```python
from build123d import *

# Parameters (mm, degrees)
F0_R      = 30
F0_R_2    = 1.55
F0_W      = 15
F0_H      = 3.2
F1_DEPTH  = 7
F3_R      = 1.6
F4_DEPTH  = 3.5
F7_COUNT  = 3
F8_R      = 5
F9_DEPTH  = 25
F11_DEPTH = 5


with BuildPart() as f1:
    # F0 (on Top) → F1 (new body)
    with BuildSketch(Plane.XY):
        Circle(F0_R)
        Polygon((-4.1143593539, -10.3262794416), (-11.6143593539, -23.3166604984), (-14.3856406461, -21.7166604984), (-6.8856406461, -8.7262794416), align=None, mode=Mode.SUBTRACT)
        with Locations((13, -22.5166604984)):
            Circle(F0_R_2, mode=Mode.SUBTRACT)
        with Locations((-26, 0)):
            Circle(F0_R_2, mode=Mode.SUBTRACT)
        Polygon((-6.8856406461, 8.7262794416), (-14.3856406461, 21.7166604984), (-11.6143593539, 23.3166604984), (-4.1143593539, 10.3262794416), align=None, mode=Mode.SUBTRACT)
        with Locations((18.5, 0)):
            Rectangle(F0_W, F0_H, mode=Mode.SUBTRACT)
        with Locations((13, 22.5166604984)):
            Circle(F0_R_2, mode=Mode.SUBTRACT)
    extrude(amount=F1_DEPTH)

    # F3 (on offset) → F4 (join)
    with BuildSketch(Plane.XZ.offset(1.6)):
        Polygon((11, 7), (26, 7), (26, 12), (23.5, 12.5), (13.5, 12.5), (11, 12), align=None)
        with Locations((18.5, 9.5)):
            Circle(F3_R, mode=Mode.SUBTRACT)
    extrude(amount=F4_DEPTH)

    # F5: F1 across plane


with BuildPart() as f1_1:
    add(f1.part)
    add(f1.part.mirror(Plane.XZ))

    # F7: F1 ×3 about axis
    f7_axis = Axis((0, 0, 17.4874160439), (0, 0, 1))


with BuildPart() as f1_2:
    add(f1_1.part)
    for i in range(1, F7_COUNT):
        add(f1_1.part.rotate(f7_axis, i * 360 / F7_COUNT))

    # F8 (on face) → F9 (cut)
    with BuildSketch(Plane.XY.offset(7)):
        Circle(F8_R)
    extrude(amount=-F9_DEPTH, mode=Mode.SUBTRACT)

    # F10 (on face) → F11 (cut)
    with BuildSketch(Plane.XY.offset(7)):
        Polygon((-30, 5), (-30, 0), (-30, -5), (-23, -5), (-23, 0), (-23, 5), align=None)
        Polygon((11.5, -19.918584287), (7.1698729811, -22.418584287), (10.6698729811, -28.4807621135), (15, -25.9807621135), (19.3301270189, -23.4807621135), (15.8301270189, -17.418584287), align=None)
        Polygon((11.5, 19.918584287), (15.8301270189, 17.418584287), (19.3301270189, 23.4807621135), (15, 25.9807621135), (10.6698729811, 28.4807621135), (7.1698729811, 22.418584287), align=None)
    extrude(amount=-F11_DEPTH, mode=Mode.SUBTRACT)


solid = f1_2.part
```
Could you check a few things on this model? Use its own coordinates, in mm. A direction names the side the tool comes from. Give positions to 0.01 mm unless a question says otherwise; leave off trailing zeros. Order: outer loops, then holes, each group sorted by start corner. A loop starts at its lowest first (then second) coordinate and runs counter-clockwise, first axis right, second up.
Q1. For faces 1 (the flat face through (18, 1.6, 6)), 2 (the flat face through (-15.88, -20.854, 9.465)), 3 (the flat face through (-26, -5, 5)), 4 (the flat face through (26, 3, 9)), which set-ups out of +Z, -Z, +X, -X, +Y, -Y let a thin tool reach every point of the face, with its end or its side?
Q2. If I drill on line 1 along Y through (x, z) = (0, 4); line 2 along Y through (x, z) = (7.5, 2.75); line 3 along Y through (x, z) = (-7.5, 10.25), over which ranges is the centre line in solid material (lowest first)?
Q3. Suppose I cut it at B-B, the plane z = 5.5. Write out the boundary of the cut face in (x, y), and give its area (3 significant figures).
Q4. We'd pull the mould along Y, two halves only. Please class faces 5 (the flat face through (-9.504, 23.112, 12.246)), 6 (the flat face through (19, -3, 12.5)), 7 (the flat face through (-9.504, -23.112, 12.246)), 8 (the flat face through (11.439, 19.954, 4.535)): +Y half, -Y half, draft (parallel to the pull), parting line (faces both ways), or undercut.
Q5. I'm going to push flat-ended pins straight in: P1, Ø1.5, axis at x = -26.5, z = 4, coming from the +Y side; P2, Ø1.9, axis at x = 13, y = -22.52, coming from the +Z side; P3, Ø6, axis at y = 16.5, z = 2.5, coming from the +X side; P4, Ø1.5, axis at x = -25.5, z = 5.5, coming from the -Y side. Where does each tip first touch, or does it pass through?
Q6. Suppose I cut it at D-D, the plane z = 1. Write out the boundary of the cut face in (x, y).
Q7. Suppose I cut it at A-A, the plane y = 0. Write out the boundary of the cut face in (x, z), and give its area (3 significant figures).
Q8. Suppose I cut it at C-C, the plane x = 0. Write out the boundary of the cut face in (y, z).
Solution:
1. face 1: +Z, -Z
1. face 2: +Z, -X, -Y
1. face 3: +Z, -X
1. face 4: +Z, +X, +Y, -Y
2. line 1: y = -30 to -5, 5 to 30
2. line 2: y = -29.05 to -22.99, -22.23 to 22.23, 22.99 to 29.05
2. line 3: y = -23.19 to -18.66, -9.79 to -8.37, 8.37 to 9.79, 18.66 to 23.19
3. outline: (-29.58, -5) arc R30 ccw to (10.46, -28.12) - (7.17, -22.42) - (15.83, -17.42) - (19.12, -23.12) arc R30 ccw to (19.12, 23.12) - (15.83, 17.42) - (7.17, 22.42) - (10.46, 28.12) arc R30 ccw to (-29.58, 5) - (-23, 5) - (-23, -5) - close; hole (-14.39, -21.72) - (-11.61, -23.32) - (-4.11, -10.33) - (-6.89, -8.73) - close; hole (-14.39, 21.72) - (-6.89, 8.73) - (-4.11, 10.33) - (-11.61, 23.32) - close; hole circle Ø10 at (0, 0); hole (11, -1.6) - (26, -1.6) - (26, 1.6) - (11, 1.6) - close
3. area: 2,400 mm2
4. face 5: +Y half
4. face 6: draft
4. face 7: -Y half
4. face 8: undercut
5. P1: stops at y = 15.39
5. P2: passes through
5. P3: stops at x = 26.79
5. P4: stops at y = -16.95
6. outline: circle Ø60 at (0, 0); hole circle Ø3.1 at (-26, 0); hole (-14.39, -21.72) - (-11.61, -23.32) - (-4.11, -10.33) - (-6.89, -8.73) - close; hole (-14.39, 21.72) - (-6.89, 8.73) - (-4.11, 10.33) - (-11.61, 23.32) - close; hole circle Ø10 at (0, 0); hole (11, -1.6) - (26, -1.6) - (26, 1.6) - (11, 1.6) - close; hole circle Ø3.1 at (13, -22.52); hole circle Ø3.1 at (13, 22.52)
7. outline: (-30, 0) - (-27.55, 0) - (-27.55, 2) - (-30, 2) - close; (-24.45, 0) - (-5, 0) - (-5, 7) - (-23, 7) - (-23, 2) - (-24.45, 2) - close; (5, 0) - (11, 0) - (11, 7) - (5, 7) - close; (26, 0) - (30, 0) - (30, 7) - (26, 7) - close
7. area: 204 mm2
8. outline: (-30, 0) - (-5, 0) - (-5, 7) - (-30, 7) - close; (5, 0) - (30, 0) - (30, 7) - (5, 7) - close
